```python
from build123d import *

# Parameters (mm, degrees)
ESQUISSE1_R               = 6
BOSS_EXTRU_1_DEPTH        = 104
TROU_TARAUD_M5X0_81_D     = 4.2
TROU_TARAUD_M5X0_81_DEPTH = 20
TROU_TARAUD_M5X0_81_TIP   = 1.2618073
TROU_TARAUD_M5X0_82_D     = 4.2
TROU_TARAUD_M5X0_82_DEPTH = 20
TROU_TARAUD_M5X0_82_TIP   = 1.2618073
CHANFREIN1_SIZE           = 0.5


with BuildPart() as part:
    # Esquisse1 → Boss.-Extru.1 (new body)
    with BuildSketch(Plane.XY):
        Circle(ESQUISSE1_R)
    extrude(amount=BOSS_EXTRU_1_DEPTH)

    # Trou taraudé M5x0.81
    with Locations(Plane(origin=(0, 0, 0), x_dir=(-1, 0, 0), z_dir=(0, 0, -1))):
        with Locations((0, 0)):
            Hole(TROU_TARAUD_M5X0_81_D / 2, depth=TROU_TARAUD_M5X0_81_DEPTH)
            with Locations((0, 0, -(TROU_TARAUD_M5X0_81_DEPTH + TROU_TARAUD_M5X0_81_TIP / 2))):  # 118° drill point
                Cone(0, TROU_TARAUD_M5X0_81_D / 2, TROU_TARAUD_M5X0_81_TIP, mode=Mode.SUBTRACT)

    # Trou taraudé M5x0.82
    with Locations(Plane.XY.offset(104)):
        with Locations((0, 0)):
            Hole(TROU_TARAUD_M5X0_82_D / 2, depth=TROU_TARAUD_M5X0_82_DEPTH)
            with Locations((0, 0, -(TROU_TARAUD_M5X0_82_DEPTH + TROU_TARAUD_M5X0_82_TIP / 2))):  # 118° drill point
                Cone(0, TROU_TARAUD_M5X0_82_D / 2, TROU_TARAUD_M5X0_82_TIP, mode=Mode.SUBTRACT)

    # Chanfrein1
    chanfrein1_edges = [part.edges().sort_by_distance(p)[0] for p in [
        (-6, 0, 0),
        (-6, 0, 104),
    ]]
    chamfer(chanfrein1_edges, length=CHANFREIN1_SIZE)


solid = part.part
```
For this review, take the finished solid that the model builds, in its own axes (mm). A direction names the side the tool comes from. Coordinates: 2 decimals unless noted, no trailing zeros. Write each loop counter-clockwise with the first axis right and the second up, starting at its lowest first coordinate (ties: lowest second). Pieces come first, ordered by that corner, then holes. Notation, with made-up numbers: (83.5, 62.25) -> (131.5, 62.25) arc R17 cw to (131.5, 93.25) -> close; hole circle Ø5 at (-17.75, 31.5). An arc over 180 degrees is marked (long way). Put each result on its own line as item: value.
Q1. The part is to be moulded in two halves that separate along X. For faces 1 (the cylindrical face through (-2.003, 0.631, 93.86)), 2 (the cylindrical face through (-6, 0, 51)), 3 (the conical face through (0.35, 0.11, 82.96)), 4 (the flat face through (-0.1, -2.4, 104)), say which applies: +X half, -X half, draft (parallel to the pull), parting line (faces both ways), or undercut.
From the geometry:
face 1: undercut
face 2: parting line
face 3: undercut
face 4: draft
Q2. Take a section at B-B, the plane z = 16.5. State the section outline as (x, y) points, then the cut area to 3 significant figures.
From the geometry:
outline: circle Ø12 at (0, 0); hole circle Ø4.2 at (0, 0)
area: 99.2 mm2
Q3. Take a section at A-A, the plane z = 47.5. State the section outline as (x, y) points.
From the geometry:
outline: circle Ø12 at (0, 0)
Q4. Wall thickness on L1, parallel to Y at x = 0, z = 5.5; L2, parallel to X at y = 0.5, z = 69; L3, parallel to Y at x = -3.75, z = 87: over which ranges is each line inside the solid? List them lowest first.
From the geometry:
L1: y = -6 to -2.1, 2.1 to 6
L2: x = -5.98 to 5.98
L3: y = -4.68 to 4.68
Q5. Tool access review of faces 5 (the flat face through (-0.1, -2.4, 0)), 6 (the cylindrical face through (2.003, 0.631, 10.14)): name each direction out of +Z, -Z, +X, -X, +Y, -Y from which nothing blocks a thin tool from reaching the whole face with its end or side.
From the geometry:
face 5: -Z, +X, -X, +Y, -Y
face 6: -Z
Q6. Clearance check with flat-ended pins moving along their axes: pin 1 Ø6 at (x, z) = (-5, 76) entering from +Y; pin 2 Ø5 at (y, z) = (-2.5, 28.5) entering from +X; pin 3 Ø4 at (x, y) = (0, 0) entering from -Z; pin 4 Ø2.5 at (x, y) = (0, 0) entering from -Z. State where each tip first meets the part, or that it passes through.
From the geometry:
pin 1: stops at y = 5.66
pin 2: stops at x = 6
pin 3: stops at z = 20.06
pin 4: stops at z = 20.51
